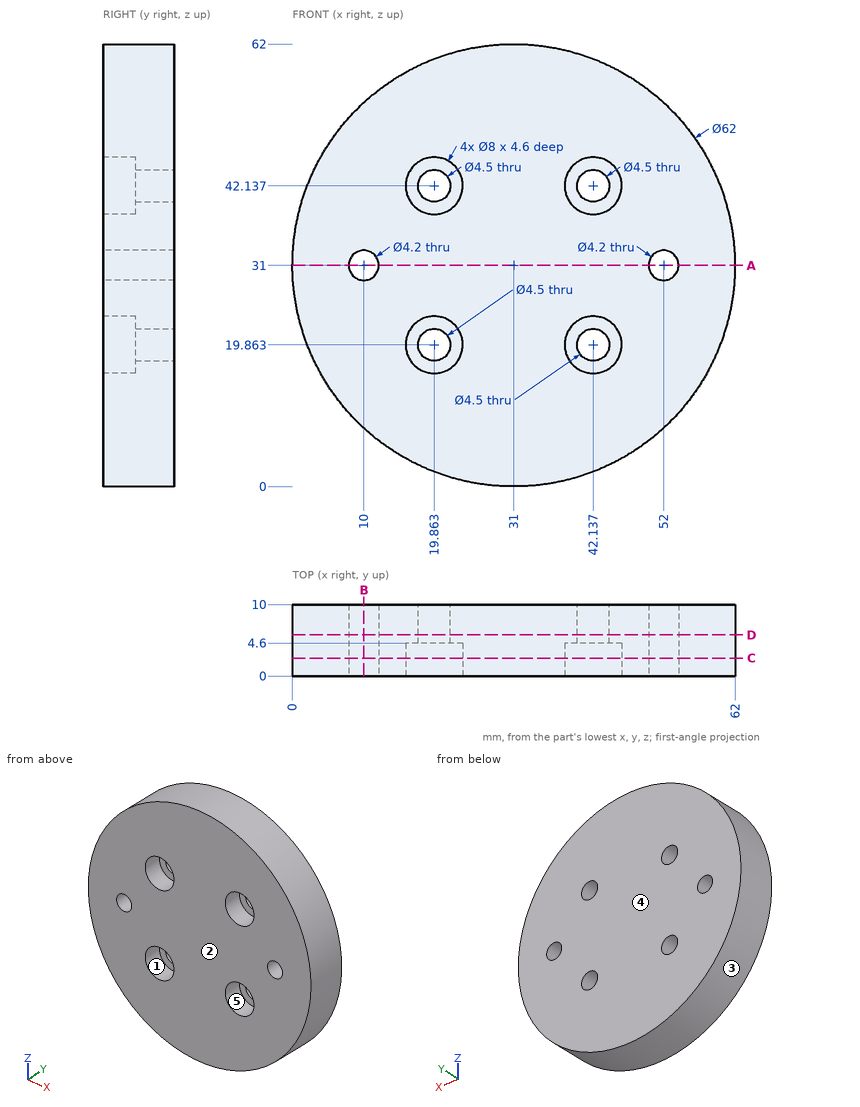
Source: three-view drawing plus pictorial views. Frame: mm from the lowest corner of the part. A direction names the side the tool comes from. Coordinates: 2 decimals unless noted, no trailing zeros. Order: outer loops, then holes, each group sorted by start corner. A loop starts at its lowest first (then second) coordinate and runs counter-clockwise, first axis right, second up. Notation, with made-up numbers: M 7,73.25 L 27,73.25 A27 cw 27,100.25 Z; hole C 6,57.25 d2. An arc over 180 degrees is marked long. Write each question's results on one line, items separated by ' | '. Start each with the question number.
1. Section C-C, the plane y = 2.5. Return the cut outline in (x, z).
2. Draft query along X for the marked faces 1, 2 and 3. Return one class per face: +X half, -X half, draft (parallel to the pull), parting line (faces both ways), or undercut.
3. Section A-A, the plane z = 31. Return the cut outline in (x, y), then the cut area to 3 significant figures.
4. Reachability of the marked faces 4 and 5 from +Z, -Z, +X, -X, +Y, -Y: full face, straight path, thin tool, end or side. Return the list, or none.
5. Material intervals for L1, parallel to X at y = 0.5, z = 42; L2, parallel to X at y = 9, z = 42; L3, parallel to X at y = 3.5, z = 56, sorted ascending.
6. Pin query (flat end, axial travel): pin 1 (6.5 mm diameter, centred on x = 21.5, z = 43, fed in from -Y); pin 2 (1 mm diameter, centred on x = 32, y = 3.5, fed in from +Z); pin 3 (1.5 mm diameter, centred on y = 8.5, z = 26.5, fed in from -X); pin 4 (1 mm diameter, centred on y = 2.5, z = 26.5, fed in from +X). Return the tip coordinate at first contact, or that it passes through.
7. Section D-D, the plane y = 5.75. Return the cut outline in (x, z), then the cut area to 3 significant figures.
8. Section B-B, the plane x = 10. Return the cut outline in (y, z).
Solution:
1) outline: C 31,31 d62; hole C 10,31 d4.2; hole C 19.86,19.86 d8; hole C 19.86,42.14 d8; hole C 42.14,19.86 d8; hole C 42.14,42.14 d8; hole C 52,31 d4.2
2) face 1: undercut | face 2: draft | face 3: parting line
3) outline: M 0,0 L 7.9,0 L 7.9,10 L 0,10 Z; M 12.1,0 L 49.9,0 L 49.9,10 L 12.1,10 Z; M 54.1,0 L 62,0 L 62,10 L 54.1,10 Z | area: 536 mm²
4) face 4: +Z, -Z, +X, -X, +Y | face 5: -Y
5) L1: 2.02 to 15.87, 23.86 to 38.14, 46.13 to 59.98 | L2: 2.02 to 17.62, 22.11 to 39.89, 44.38 to 59.98 | L3: 12.67 to 49.33
6) pin 1: y = 0 | pin 2: z = 62 | pin 3: x = 0.23 | pin 4: x = 61.74
7) outline: C 31,31 d62; hole C 10,31 d4.2; hole C 19.86,19.86 d4.5; hole C 19.86,42.14 d4.5; hole C 42.14,19.86 d4.5; hole C 42.14,42.14 d4.5; hole C 52,31 d4.2 | area: 2,930 mm²
8) outline: M 0,8.2 L 10,8.2 L 10,28.9 L 0,28.9 Z; M 0,33.1 L 10,33.1 L 10,53.8 L 0,53.8 Z
